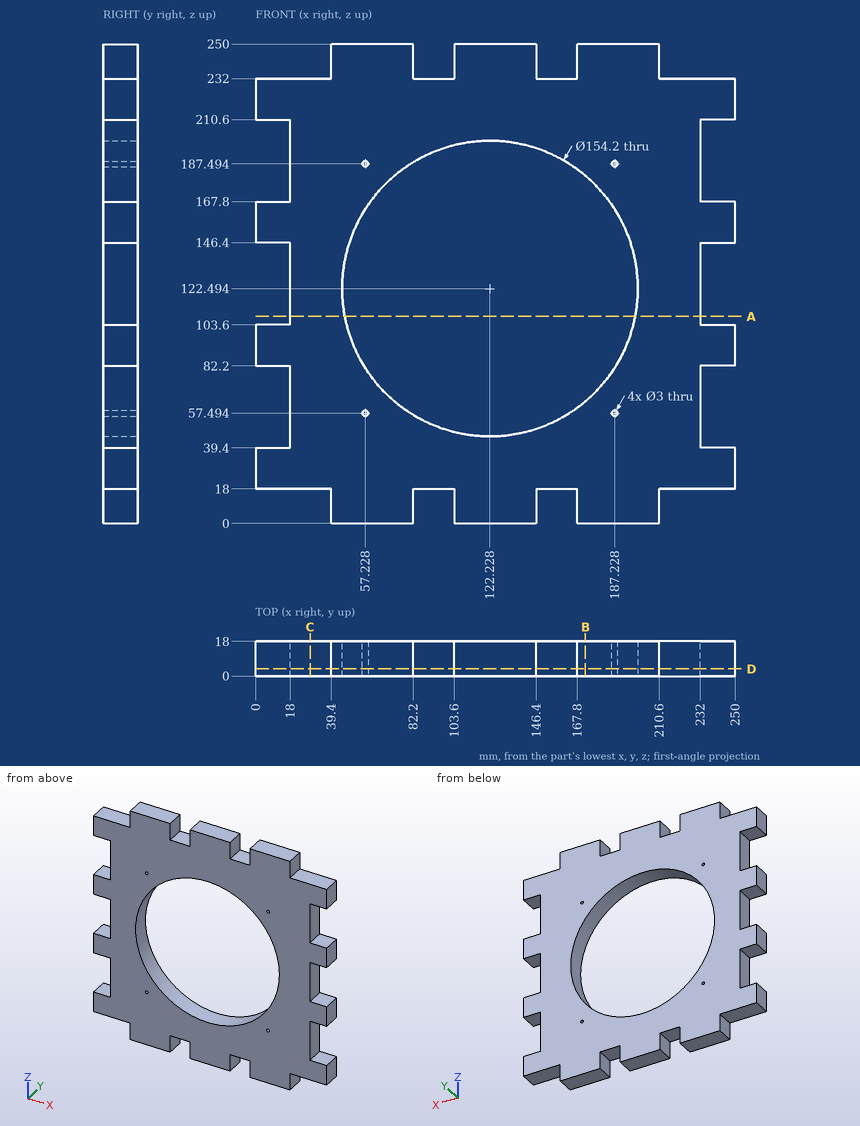
Can you work these out from the drawing? Everything is in mm from the part's minimum corner. Coordinates: 2 decimals unless noted, no trailing zeros. Write each loop counter-clockwise with the first axis right and the second up, starting at its lowest first coordinate (ties: lowest second). Pieces come first, ordered by that corner, then holes. Notation, with made-up numbers: (-38.5, -6) -> (-6.5, -6) arc R17 cw to (-6.5, 5) -> close; hole circle Ø7 at (-34, 76). An arc over 180 degrees is marked (long way). Write each question's results on one line, items separated by ' | '. Start each with the question number.
Item 1: If we section it at D-D, the plane y = 3.75: Count the separate pieces of the cut face and the enclosed holes in it, and give its area (3 significant figures).
Item 2: If we section it at A-A, the plane z = 108: Write out the boundary of the cut face in (x, y).
Item 3: If we section it at B-B, the plane x = 172: Write out the boundary of the cut face in (y, z).
Item 4: I'm going to push flat-ended pins straight in: P1, Ø9, axis at x = 152.5, y = 12.5, coming from the -Z side; P2, Ø2, axis at y = 11, z = 42, coming from the -X side; P3, Ø9, axis at y = 6.5, z = 54.5, coming from the +X side. Where does each tip first touch, or does it pass through?
Item 5: If we section it at C-C, the plane x = 28.5: Write out the boundary of the cut face in (y, z), and give its area (3 significant figures).
Item 6: Please list where these lines run through material, in increasing order: probe 1 along Z at (x, y) = (16, 7); probe 2 along Z at (x, y) = (124.5, 3.75); probe 3 along Z at (x, y) = (224, 4.75).
Answer block:
1) separate pieces: 1 | enclosed holes: 5 | area: 34,800 mm²
2) outline: (18, 0) -> (46.5, 0) -> (46.5, 18) -> (18, 18) -> close; (197.95, 0) -> (232, 0) -> (232, 18) -> (197.95, 18) -> close
3) outline: (0, 0) -> (18, 0) -> (18, 63.61) -> (0, 63.61) -> close; (0, 181.38) -> (18, 181.38) -> (18, 250) -> (0, 250) -> close
4) P1: z = 18 | P2: x = 18 | P3: x = 232
5) outline: (0, 18) -> (18, 18) -> (18, 232) -> (0, 232) -> close | area: 3,850 mm²
6) probe 1: 18 to 39.4, 82.2 to 103.6, 146.4 to 167.8, 210.6 to 232 | probe 2: 0 to 45.43, 199.56 to 250 | probe 3: 18 to 232
